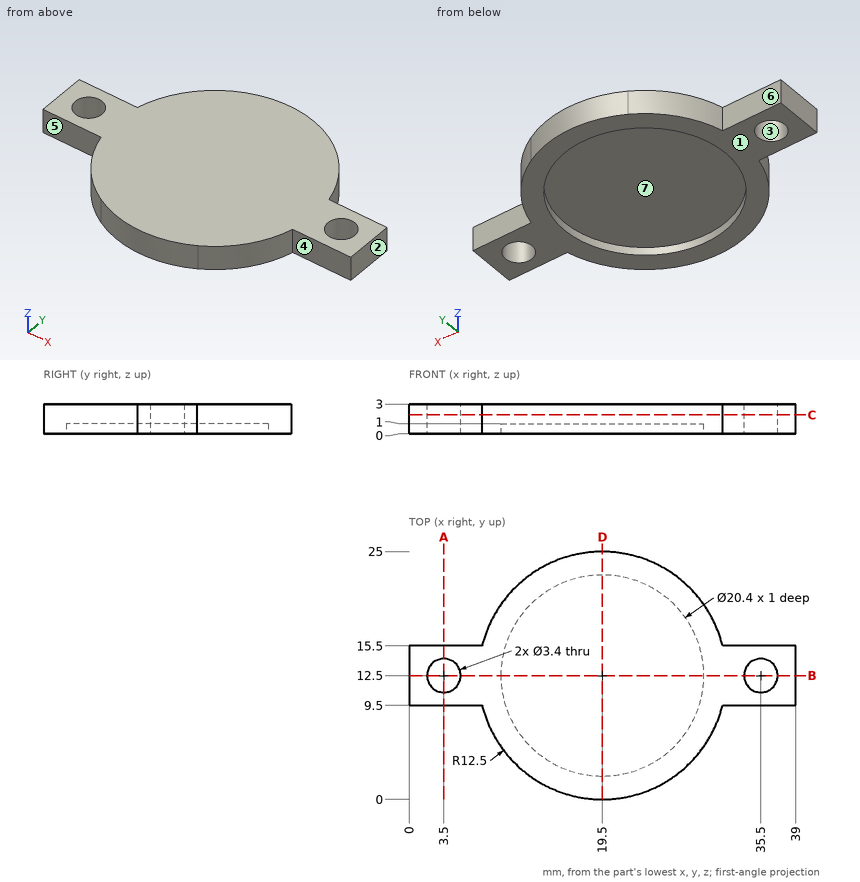
Design review of the part shown in the three views and the two pictorial views. Dimensions are in mm from the part's minimum x, y and z. A direction names the side the tool comes from. Coordinates: 2 decimals unless noted, no trailing zeros. Order: outer loops, then holes, each group sorted by start corner. A loop starts at its lowest first (then second) coordinate and runs counter-clockwise, first axis right, second up. Notation, with made-up numbers: (18.25, -14) - (34.25, -14) arc R14 cw to (34.25, 13) - close; hole circle Ø5 at (31.5, 3). An arc over 180 degrees is marked (long way). Answer as CSV lines item,"result". Start each with the question number.
1) Add section C-C (z = 1.9). State the section outline as (x, y) points.
2) Insertion check: P1, Ø1, axis at x = 18, z = 2.5, coming from the +Y side; P2, Ø0.9, axis at x = 37, z = 2, coming from the +Y side; P3, Ø1.5, axis at x = 14.5, z = 2, coming from the +Y side. Each pin has a flat end and moves straight along its axis. Give the tip position at first contact, or say it passes through.
3) Machinability: for the marked faces 4, 5, 6 and 7, which of the approach directions +Z, -Z, +X, -X, +Y, -Y give a long, thin tool a straight path to every point of the face, cutting with its end or side? Answer none if there is none.
4) Draft analysis for pull direction X (two halves, no side actions). For the marked faces 1, 2 and 3, state which applies: +X half, -X half, draft (parallel to the pull), parting line (faces both ways), or undercut.
5) Add section B-B (y = 12.5). State the section outline as (x, z) points, then the cut area to 3 significant figures.
6) Add section A-A (x = 3.5). State the section outline as (y, z) points, then the cut area to 3 significant figures.
7) Add section D-D (x = 19.5). State the section outline as (y, z) points, then the cut area to 3 significant figures.
8) To check wall thickness, follow line 1 along Y through (x, z) = (35.5, 2.2); line 2 along Y through (x, z) = (19.5, 0.5); line 3 along Z through (x, y) = (12, 16). State the ranges of each line that lie inside material, in increasing order. Write a range as [from, to].
Result:
1,outline,"(0, 9.5) - (7.37, 9.5) arc R12.5 ccw to (31.63, 9.5) - (39, 9.5) - (39, 15.5) - (31.63, 15.5) arc R12.5 ccw to (7.37, 15.5) - (0, 15.5) - close; hole circle Ø3.4 at (3.5, 12.5); hole circle Ø3.4 at (35.5, 12.5)"
2,P1,"y = 24.96"
2,P2,"y = 15.5"
2,P3,"y = 24.26"
3,face 4,"+Z, -Z, +X, -Y"
3,face 5,"+Z, -Z, -X, -Y"
3,face 6,"+Z, -Z, -X, +Y"
3,face 7,"-Z"
4,face 1,"draft"
4,face 2,"+X half"
4,face 3,"undercut"
5,outline,"(0, 0) - (1.8, 0) - (1.8, 3) - (0, 3) - close; (5.2, 0) - (9.3, 0) - (9.3, 1) - (29.7, 1) - (29.7, 0) - (33.8, 0) - (33.8, 3) - (5.2, 3) - close; (37.2, 0) - (39, 0) - (39, 3) - (37.2, 3) - close"
5,area,"76.2 mm^2"
6,outline,"(9.5, 0) - (10.8, 0) - (10.8, 3) - (9.5, 3) - close; (14.2, 0) - (15.5, 0) - (15.5, 3) - (14.2, 3) - close"
6,area,"7.80 mm^2"
7,outline,"(0, 0) - (2.3, 0) - (2.3, 1) - (22.7, 1) - (22.7, 0) - (25, 0) - (25, 3) - (0, 3) - close"
7,area,"54.6 mm^2"
8,line 1,"[9.5, 10.8], [14.2, 15.5]"
8,line 2,"[0, 2.3], [22.7, 25]"
8,line 3,"[1, 3]"
